Solid Edge part; units mm, degrees
sketch "Sketch1" plane through (0, 0, 0) normal (0, 0, 1) x (1, 0, 0)
  circle A0 centre (0, 0) radius 1.6
extrude "Protrusion1" add sketch "Sketch1" against normal blind 6
sketch "Sketch2" plane through (0, 0, 0) normal (0, 0, 1) x (1, 0, 0)
  circle A0 centre (0, 0) radius 2
extrude "ExtrudedProtrusion_2" add sketch "Sketch2" along normal blind 0.25
sketch "Sketch3" plane through (0, 0, 0) normal (0, -1, 0) x (1, 0, 0)
  line L0 (0.1, 0.125) -> (0.1, 0.25)
  line L1 (0.1, 0.25) -> (-0.1, 0.25)
  line L2 (-0.1, 0.25) -> (-0.1, 0.125)
  line L3 (-0.1, 0.125) -> (0.1, 0.125)
extrude "Cutout1" cut sketch "Sketch3" against normal up to next
sketch "Sketch4" plane through (0, 0, 0) normal (0, -1, 0) x (1, 0, 0)
  line L0 (0.1, 0.25) -> (-0.1, 0.25)
  line L1 (-0.1, 0.25) -> (-0.1, 0.125)
  line L2 (-0.1, 0.125) -> (0.1, 0.125)
  line L3 (0.1, 0.125) -> (0.1, 0.25)
extrude "Cutout2" cut sketch "Sketch4" along normal up to next
Can you work these out from the model? Positions are in its coordinate system, mm. A direction names the side the tool comes from. Round coordinates to 2 decimals unless told otherwise and drop trailing zeros. Loops run counter-clockwise (first coordinate to the right, second up) from the corner with the lowest first, then second, coordinate; pieces in that order, holes last. Notation, with made-up numbers: (71, 70.5) - (123, 70.5) arc R22 cw to (123, 103.5) - close; hole circle Ø4 at (-2, 1.25). An arc over 180 degrees is marked (long way). Answer in a Markdown table with one row per item. Add a question column.
Q1. I need wall thicknesses on L1, parallel to Y at x = 0.05, z = -1.25; L2, parallel to Z at x = 1.6, y = 0.65; L3, parallel to X at y = -1.4, z = -4. Which ranges of each line are inside material? Lowest first, please.
Q2. I want a section at D-D on x = -1.25. List the corners of the cut face in (y, z) for me, and give its area (3 significant figures).
Q3. I want a section at C-C on z = -2.5. List the corners of the cut face in (x, y) for me, and give its area (3 significant figures).
Q4. Which directions (+Z, -Z, +X, -X, +Y, -Y) give clear straight access to the entire face, cutting with the end or side of a thin tool? Please do faces 1 (the cylindrical face through (-1.27, -0.97, -2.96)), 2 (the flat face through (0, 0, -6)).
Q5. I want a section at A-A on y = 0. List the corners of the cut face in (x, z) for me (3 decimals), and give its area (3 significant figures).
Q6. I want a section at B-B on x = 0. List the corners of the cut face in (y, z) for me (3 decimals).
A:
| question | item | result |
|---|---|---|
| 1 | L1 | -1.6 to 1.6 |
| 1 | L2 | 0 to 0.25 |
| 1 | L3 | -0.77 to 0.77 |
| 2 | outline | (-1.56, 0) - (-1, 0) - (-1, -6) - (1, -6) - (1, 0) - (1.56, 0) - (1.56, 0.25) - (-1.56, 0.25) - close |
| 2 | area | 12.8 mm^2 |
| 3 | outline | circle Ø3.2 at (0, 0) |
| 3 | area | 8.04 mm^2 |
| 4 | face 1 | -Z |
| 4 | face 2 | -Z, +X, -X, +Y, -Y |
| 5 | outline | (-2, 0) - (-1.6, 0) - (-1.6, -6) - (1.6, -6) - (1.6, 0) - (2, 0) - (2, 0.25) - (0.1, 0.25) - (0.1, 0.125) - (-0.1, 0.125) - (-0.1, 0.25) - (-2, 0.25) - close |
| 5 | area | 20.2 mm^2 |
| 6 | outline | (-2, 0) - (-1.6, 0) - (-1.6, -6) - (1.6, -6) - (1.6, 0) - (2, 0) - (2, 0.125) - (-2, 0.125) - close |
